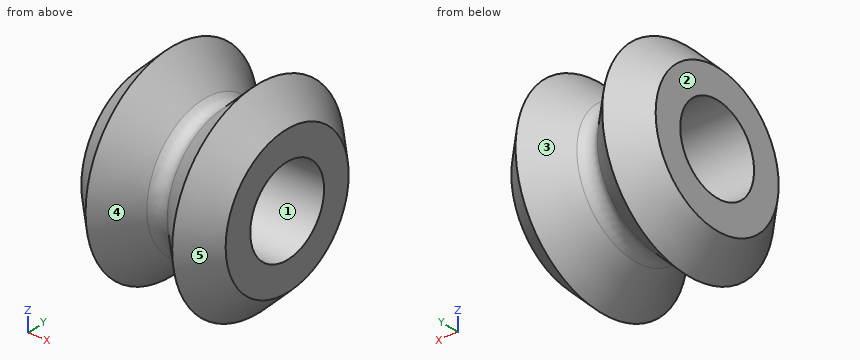
```python
from build123d import *

# Parameters (mm, degrees)
FILLET1_R          = 1
SKETCH2_R          = 3
CUT_EXTRUDE1_DEPTH = 15.071247379


with BuildPart() as part:
    # Sketch1 → Revolve1 (revolve)
    with BuildSketch(Plane.XY, mode=Mode.PRIVATE) as revolve1_sk:
        Polygon((5, 0), (5, 5), (3, 7), (0, 4), (-3, 7), (-5, 5), (-5, 0), align=None)
    revolve(revolve1_sk.sketch.rotate(Axis((-5, 0, 0), (1, 0, 0)), 180), axis=Axis((-5, 0, 0), (1, 0, 0)))

    # Fillet1
    fillet1_edges = [part.edges().sort_by_distance(p)[0] for p in [
        (0, 4, 0),
    ]]
    fillet(fillet1_edges, radius=FILLET1_R)

    # Sketch2 → Cut-Extrude1 (cut, through all)
    with BuildSketch(Plane(origin=(5, 0, 0), x_dir=(0, 0, -1), z_dir=(1, 0, 0))):
        with Locations(Location((0, 0, 0), (0, 0, 90))):
            Circle(SKETCH2_R)
    extrude(amount=-CUT_EXTRUDE1_DEPTH, mode=Mode.SUBTRACT)


solid = part.part
```
CAD build for the part. Positions are in the model's coordinates, mm. Face numbers are marked on the shaded views. A direction names the side the tool comes from. Round coordinates to 2 decimals unless told otherwise and drop trailing zeros. Order: outer loops, then holes, each group sorted by start corner. A loop starts at its lowest first (then second) coordinate and runs counter-clockwise, first axis right, second up. Notation, with made-up numbers: (71.25, 45) - (101.25, 45) arc R17 ccw to (101.25, 58) - close; hole circle Ø1 at (21.25, -11). An arc over 180 degrees is marked (long way). Answer in a Markdown table with one row per item. Add a question column.
(1) Band-saw the part on A-A on x = -1. List the corners of the cut face in (y, z), and give its area (3 significant figures).
(2) 3-axis set-ups, long thin cutter, end or side, ignore diameter. For the marked faces 4 and 5: which of +Z, -Z, +X, -X, +Y, -Y reach the whole face in a straight line?
(3) Drop flat-ended pins along their axis: pin 1 Ø2 at (y, z) = (-0.5, -1) entering from +X; pin 2 Ø4 at (x, z) = (-0.5, -5) entering from -Y. Give the stop position or say it passes through.
(4) Probe L1, parallel to Z at x = 1, y = 0; L2, parallel to Z at x = -2, y = 0; L3, parallel to X at y = 3.75, z = 3.25. List the from-to ranges inside material, lowest first. Write a range as [from, to].
(5) Band-saw the part on B-B on x = 2.25. List the corners of the cut face in (y, z).
(6) Mould opens along Z. For the marked faces 1, 2 and 3 say: +Z half, -Z half, draft (parallel to the pull), parting line (faces both ways), or undercut.
Data:
| question | item | result |
|---|---|---|
| 1 | outline | circle Ø10 at (0, 0); hole circle Ø6 at (0, 0) |
| 1 | area | 50.3 mm^2 |
| 2 | face 4 | none |
| 2 | face 5 | +X |
| 3 | pin 1 | passes through |
| 3 | pin 2 | stops at y = -4.78 |
| 4 | L1 | z = [-5, -3], [3, 5] |
| 4 | L2 | z = [-6, -3], [3, 6] |
| 4 | L3 | x = [-5, -0.96], [0.96, 5] |
| 5 | outline | circle Ø12.5 at (0, 0); hole circle Ø6 at (0, 0) |
| 6 | face 1 | undercut |
| 6 | face 2 | draft |
| 6 | face 3 | parting line |
